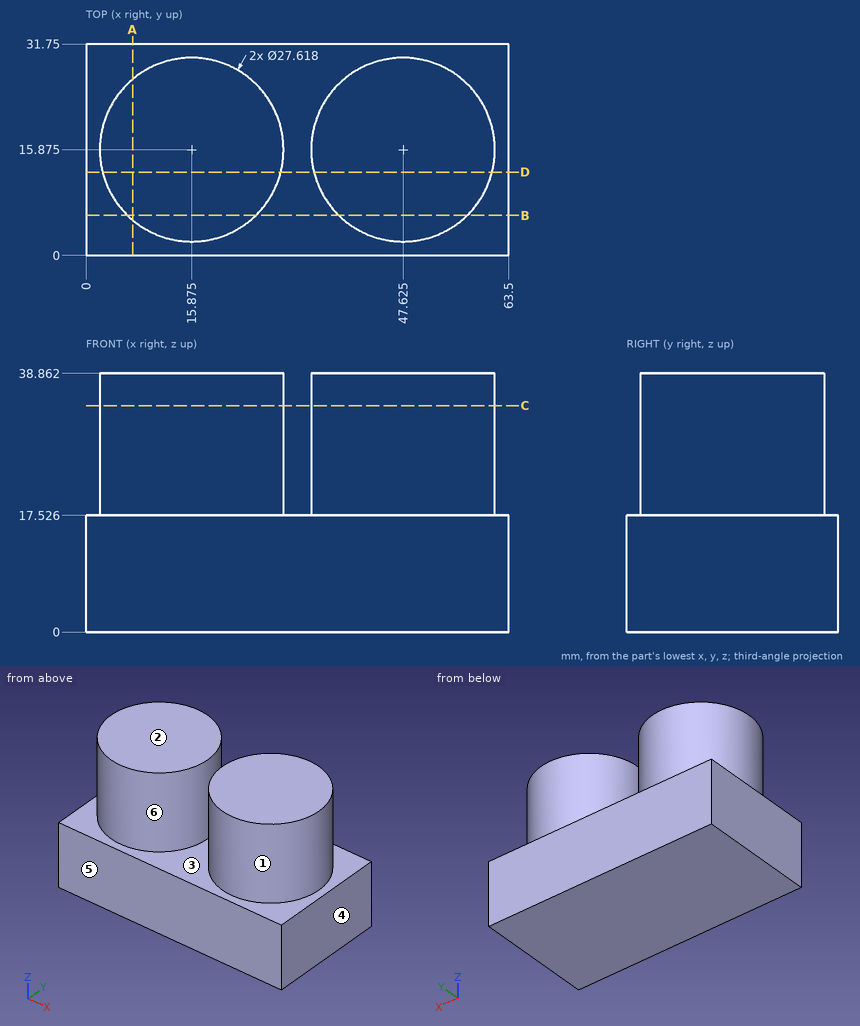
Design review of the part shown in the three views and the two pictorial views. Dimensions are in mm from the part's minimum x, y and z. A direction names the side the tool comes from. Give positions to 0.01 mm unless a question says otherwise; leave off trailing zeros. Order: outer loops, then holes, each group sorted by start corner. A loop starts at its lowest first (then second) coordinate and runs counter-clockwise, first axis right, second up. Notation, with made-up numbers: M 17.5,27 L 21.5,27 A23 cw 21.5,35 Z; hole C 48.5,5.5 d8. An arc over 180 degrees is marked long. Answer in a Markdown table with one row per item. Add a question column.
(1) Wall thickness on probe 1 along Z at (x, y) = (33, 20.5); probe 2 along X at (y, z) = (13, 30.5); probe 3 along X at (y, z) = (14, 26): over which ranges is each line inside the solid? List them lowest first. Write a range as [from, to].
(2) For the marked faces 5 and 6, list the 3-axis set-ups (+Z, -Z, +X, -X, +Y, -Y) from which the entire face can be reached by the end or side of a thin tool; tool diameter is ignored.
(3) Consider section A-A on x = 7. State the section outline as (y, z) points, and give its area (3 significant figures).
(4) Consider section D-D on y = 12.5. State the section outline as (x, z) points (3 decimals).
(5) Consider section B-B on y = 6. State the section outline as (x, z) points, and give its area (3 significant figures).
(6) For pin 1 (10 mm diameter, centred on x = 49.5, y = 6, fed in from -Z); pin 2 (8 mm diameter, centred on y = 5.5, z = 33, fed in from -X); pin 3 (1.5 mm diameter, centred on x = 14, z = 31, fed in from +Y); pin 4 (4 mm diameter, centred on x = 13.5, z = 33.5, fed in from -Y), all flat-tipped, find the tip position at first contact; note any pin that passes through.
(7) Consider section C-C on z = 34. State the section outline as (x, y) points (3 decimals), and give its area (3 significant figures).
(8) Mouldability with a two-part tool opening along X and no side actions: class the marked faces 1, 2, 3 and 4 as +X half, -X half, draft (parallel to the pull), parting line (faces both ways), or undercut.
Evaluation:
| question | item | result |
|---|---|---|
| 1 | probe 1 | z = [0, 17.53] |
| 1 | probe 2 | x = [2.37, 29.38], [34.12, 61.13] |
| 1 | probe 3 | x = [2.19, 29.56], [33.94, 61.31] |
| 2 | face 5 | +Z, -Z, +X, -X, -Y |
| 2 | face 6 | +Z |
| 3 | outline | M 0,0 L 31.75,0 L 31.75,17.53 L 26.45,17.53 L 26.45,38.86 L 5.3,38.86 L 5.3,17.53 L 0,17.53 Z |
| 3 | area | 1,010 mm^2 |
| 4 | outline | M 0,0 L 63.5,0 L 63.5,17.526 L 61.015,17.526 L 61.015,38.862 L 34.235,38.862 L 34.235,17.526 L 29.265,17.526 L 29.265,38.862 L 2.485,38.862 L 2.485,17.526 L 0,17.526 Z |
| 5 | outline | M 0,0 L 63.5,0 L 63.5,17.53 L 57.28,17.53 L 57.28,38.86 L 37.97,38.86 L 37.97,17.53 L 25.53,17.53 L 25.53,38.86 L 6.22,38.86 L 6.22,17.53 L 0,17.53 Z |
| 5 | area | 1,940 mm^2 |
| 6 | pin 1 | stops at z = 0 |
| 6 | pin 2 | stops at x = 3.63 |
| 6 | pin 3 | stops at y = 29.64 |
| 6 | pin 4 | stops at y = 2.07 |
| 7 | outline | C 15.875,15.875 d27.618; C 47.625,15.875 d27.618 |
| 7 | area | 1,200 mm^2 |
| 8 | face 1 | undercut |
| 8 | face 2 | draft |
| 8 | face 3 | undercut |
| 8 | face 4 | +X half |
